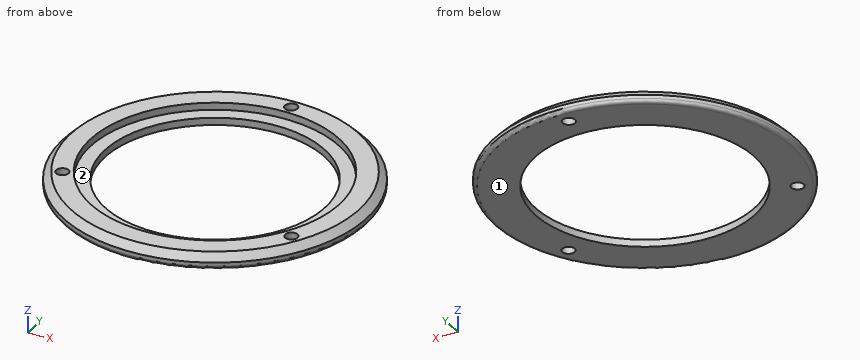
from build123d import *

# Parameters (mm, degrees)
SKETCH_1_R          = 42
SKETCH_1_R_2        = 30.5
EXTRUDE_1_DEPTH     = 4
CHAMFER_1_SIZE      = 2
SKETCH_3_R          = 34.5
CUT_EXTRUDE_2_DEPTH = 2
SKETCH_4_R          = 1.75
CUT_EXTRUDE_5_DEPTH = 60.531504265
FILLET_2_R          = 1


with BuildPart() as part:
    # Эскиз1 → Бобышка-Вытянуть1 (new body)
    with BuildSketch(Plane.XY):
        Circle(SKETCH_1_R)
        Circle(SKETCH_1_R_2, mode=Mode.SUBTRACT)
    extrude(amount=EXTRUDE_1_DEPTH)

    # Фаска1
    chamfer_1_edges = [part.edges().sort_by_distance(p)[0] for p in [
        (-42, 0, 4),
    ]]
    chamfer(chamfer_1_edges, length=CHAMFER_1_SIZE)

    # Эскиз3 → Вырез-Вытянуть2 (cut)
    with BuildSketch(Plane.XY.offset(4)):
        Circle(SKETCH_3_R)
    extrude(amount=-CUT_EXTRUDE_2_DEPTH, mode=Mode.SUBTRACT)

    # Эскиз4 → Вырез-Вытянуть5 (cut, through all)
    with BuildSketch(Plane.XY.offset(4)):
        with Locations((0, 37.25)):
            Circle(SKETCH_4_R)
        with Locations((32.259446291, -18.625)):
            Circle(SKETCH_4_R)
        with Locations((-32.259446291, -18.625)):
            Circle(SKETCH_4_R)
    extrude(amount=-CUT_EXTRUDE_5_DEPTH, mode=Mode.SUBTRACT)

    # Скругление2
    fillet_2_edges = [part.edges().sort_by_distance(p)[0] for p in [
        (-42, 0, 0),
    ]]
    fillet(fillet_2_edges, radius=FILLET_2_R)


solid = part.part
Could you check a few things on this model? Use its own coordinates, in mm. Face numbers are marked on the shaded views. Give positions to 0.01 mm unless a question says otherwise; leave off trailing zeros. Write each loop counter-clockwise with the first axis right and the second up, starting at its lowest first coordinate (ties: lowest second). Pieces come first, ordered by that corner, then holes. Notation, with made-up numbers: (29.25, 22.5) -> (79.25, 22.5) arc R24 cw to (79.25, 47.5) -> close; hole circle Ø8 at (8.5, 8). An arc over 180 degrees is marked (long way). Answer as a JSON object with one key per item and string values.
Q1. We'd pull the mould along X, two halves only. Please class the marked faces 1 and 2: released by +X, released by -X, zero draft, split by the parting line, or undercut.
Taken from the geometry:
{"face 1": "zero draft", "face 2": "undercut"}
Q2. Suppose I cut it at B-B on y = 0. Write out the boundary of the cut face in (x, z).
Taken from the geometry:
{"outline": "(-42, 1) arc R1 ccw to (-41, 0) -> (-30.5, 0) -> (-30.5, 2) -> (-34.5, 2) -> (-34.5, 4) -> (-40, 4) -> (-42, 2) -> close; (30.5, 0) -> (41, 0) arc R1 ccw to (42, 1) -> (42, 2) -> (40, 4) -> (34.5, 4) -> (34.5, 2) -> (30.5, 2) -> close"}
Q3. Suppose I cut it at A-A on x = 0. Write out the boundary of the cut face in (y, z), then the cut area to 3 significant figures.
Taken from the geometry:
{"outline": "(-42, 1) arc R1 ccw to (-41, 0) -> (-30.5, 0) -> (-30.5, 2) -> (-34.5, 2) -> (-34.5, 4) -> (-40, 4) -> (-42, 2) -> close; (30.5, 0) -> (35.5, 0) -> (35.5, 4) -> (34.5, 4) -> (34.5, 2) -> (30.5, 2) -> close; (39, 0) -> (41, 0) arc R1 ccw to (42, 1) -> (42, 2) -> (40, 4) -> (39, 4) -> close", "area": "57.6 mm²"}
Q4. Suppose I cut it at C-C on z = 3. Write out the boundary of the cut face in (x, y) (3 decimals), then the cut area to 3 significant figures.
Taken from the geometry:
{"outline": "circle Ø82 at (0, 0); hole circle Ø69 at (0, 0); hole circle Ø3.5 at (-32.259, -18.625); hole circle Ø3.5 at (0, 37.25); hole circle Ø3.5 at (32.259, -18.625)", "area": "1,510 mm²"}
Q5. Will these pins go through, and if not, where does the flat tip stop? pin 1 Ø1 at (x, z) = (-22.5, 0.5) entering from -Y; pin 2 Ø10 at (x, y) = (-22.5, -5) entering from +Z; pin 3 Ø1 at (y, z) = (-15, 1) entering from -X; pin 4 Ø5.5 at (x, y) = (0, 37.25) entering from -Z.
Taken from the geometry:
{"pin 1": "stops at y = -35.7", "pin 2": "passes through", "pin 3": "stops at x = -39.42", "pin 4": "stops at z = 0"}
Q6. Please list where these lines run through material, in increasing order: L1, parallel to Y at x = 0, z = 1.5; L2, parallel to Y at x = -31, z = 2.3; L3, parallel to Y at x = 4, z = 3.2.
Taken from the geometry:
{"L1": "y = -42 to -30.5, 30.5 to 35.5, 39 to 42", "L2": "y = -27.89 to -19.84, -17.41 to -15.14, 15.14 to 27.89", "L3": "y = -40.6 to -34.27, 34.27 to 40.6"}
